Read the model definition and answer for the solid it produces. Units are mm, in the model's axes. Give positions to 0.01 mm unless a question says otherwise; leave off trailing zeros. Order: outer loops, then holes, each group sorted by start corner. A loop starts at its lowest first (then second) coordinate and runs counter-clockwise, first axis right, second up. Notation, with made-up numbers: (18, 78.5) -> (35, 78.5) arc R19 cw to (35, 84.5) -> close; hole circle Ø9 at (7, 86). An arc over 180 degrees is marked (long way). Answer as CSV lines item,"result". Start each with the question number.
1) Find section A-A (y = 56). Determine the outline of the cut face in (x, z).
2) Straight lines are drawn through the part: L1, parallel to Y at x = -1.45, z = 13; L2, parallel to Z at x = 0.3, y = 26.5; L3, parallel to Z at x = -1.65, y = 12. For each, find the intervals that lie inside material, in ascending order. Write a range as from..to.
3) Flat-ended cylindrical pins translate along their axes: pin 1 Ø1 at (x, z) = (-0.5, 30.5) entering from -Y; pin 2 Ø1.5 at (x, z) = (-1.5, 39) entering from +Y; pin 3 Ø2 at (x, z) = (2.5, 40.5) entering from -Y. Find the tip coordinate at first contact, or state that the pin passes through.
4) Find section B-B (z = -36.5). Determine the outline of the cut face in (x, y), and give its area (3 significant figures).
```python
from build123d import *

# Parameters (mm, degrees)
SKETCH1_R                = 59
EXTRUDE1_DEPTH           = 3
EXTRUDE2_DEPTH           = 3
CIRPATTERN1_COUNT        = 6
F_2_0_2_DIAMETER_HOLE1_D = 2
F_2_0_2_DIAMETER_HOLE3_D = 2
CIRPATTERN2_COUNT        = 2
CIRPATTERN2_ANGLE        = 60


with BuildPart() as part:
    # Sketch1 → Extrude1 (new, symmetric)
    with BuildSketch(Plane(origin=(0, 0, 0), x_dir=(0, 0, -1), z_dir=(1, 0, 0))):
        Circle(SKETCH1_R)
        Polygon((16.590840947, 23.694176429), (-12.224338236, 26.215177945), (-28.815179183, 2.521001516), (-16.590840947, -23.694176429), (12.224338236, -26.215177945), (28.815179183, -2.521001516), align=None, mode=Mode.SUBTRACT)
    extrude(amount=EXTRUDE1_DEPTH, both=True)

    # Sketch2 → Extrude2 (add, symmetric)
    with BuildSketch(Plane(origin=(0, 0, 0), x_dir=(0, 0, -1), z_dir=(1, 0, 0))):
        with BuildLine():
            Line((-2, 67.961805723), (-0.262709442, 61.478149092))
            ThreePointArc((-0.262709442, 61.478149092), (-0.58620663, 59.77173183), (-2.122608272, 58.961805723))
            ThreePointArc((-2.122608272, 58.961805723), (28.679663449, 51.560419941), (51.21368579, 29.294340542))
            ThreePointArc((51.21368579, 29.294340542), (36.791707484, 48.186627241), (17.927108603, 62.644803614))
            ThreePointArc((17.927108603, 62.644803614), (8.312130826, 66.609702921), (-2, 67.961805723))
        make_face()
    extrude2 = extrude(amount=EXTRUDE2_DEPTH, both=True)

    # CirPattern1: Extrude2 ×6 about axis
    cirpattern1_axis = Axis((0, 0, 0), (1, 0, 0))
    for i in range(1, CIRPATTERN1_COUNT):
        add(extrude2.rotate(cirpattern1_axis, i * 360 / CIRPATTERN1_COUNT))

    # Ø2.0 (2) Diameter Hole1 (through all)
    with Locations(Plane(origin=(3, 0, 0), x_dir=(0, 0, -1), z_dir=(1, 0, 0))):
        with Locations((-12.224338236, 26.215177945), (16.590840947, 23.694176429), (28.815179183, -2.521001516), (12.224338236, -26.215177945), (-16.590840947, -23.694176429), (-28.815179183, 2.521001516)):
            Hole(F_2_0_2_DIAMETER_HOLE1_D / 2)

    # Ø2.0 (2) Diameter Hole3 (through all)
    with Locations(Plane(origin=(3, 0, 0), x_dir=(0, 0, -1), z_dir=(1, 0, 0))):
        with Locations((-2.287213609, 25.345792192)):
            f_2_0_2_diameter_hole3 = Hole(F_2_0_2_DIAMETER_HOLE3_D / 2)

    # CirPattern2: Ø2.0 (2) Diameter Hole3 ×2 about axis
    cirpattern2_axis = Axis((-5.5, 0, 0), (-1, 0, 0))
    for i in range(1, CIRPATTERN2_COUNT):
        add(f_2_0_2_diameter_hole3.rotate(cirpattern2_axis, i * CIRPATTERN2_ANGLE / (CIRPATTERN2_COUNT - 1)), mode=Mode.SUBTRACT)


solid = part.part
```
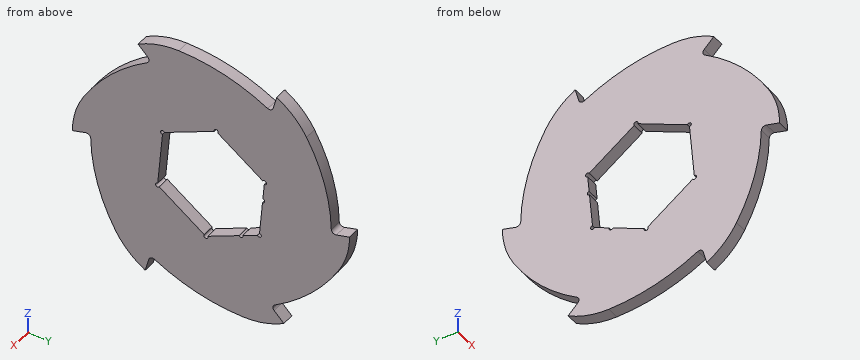
Findings below:
1,outline,"(-3, -27.89) -> (3, -27.89) -> (3, 23.17) -> (-3, 23.17) -> close"
2,L1,"-65.04..-24.01, 25.11..25.58, 26.85..58.07"
2,L2,"-61.73..11.27, 13.18..52.76"
2,L3,"-63.14..-22.04, 22.18..58.88"
3,pin 1,"y = -54.33"
3,pin 2,"y = 50.53"
3,pin 3,"y = -45.35"
4,outline,"(-3, -51.32) -> (3, -51.32) -> (3, 48.48) -> (-3, 48.48) -> close"
4,area,"599 mm²"
